Design review of the part built by this model. Coordinates are the model's own, in mm. A direction names the side the tool comes from. Coordinates: 2 decimals unless noted, no trailing zeros. Loops run counter-clockwise (first coordinate to the right, second up) from the corner with the lowest first, then second, coordinate; pieces in that order, holes last. Notation, with made-up numbers: (-40, 81) -> (12, 81) arc R15 cw to (12, 92) -> close; hole circle Ø10 at (79, 66). An arc over 180 degrees is marked (long way). Answer in a Markdown table with one row per item.
Autodesk Inventor part; units mm, degrees
ref_plane "YZ Plane" through (0, 0, 0) normal (1, 0, 0) x (0, 1, 0)
ref_plane "XZ Plane" through (0, 0, 0) normal (0, 1, 0) x (-1, 0, 0)
ref_plane "XY Plane" through (0, 0, 0) normal (0, 0, 1) x (1, 0, 0)
sketch "Sketch8" plane through (0, 0, 0) normal (1, 0, 0) x (0, 1, 0)
  line L0 (0, 15.5) -> (0, 5.5)
  line L1 (0, 5.5) -> (5, 5.5)
  line L2 (5, 5.5) -> (5, -5.5)
  line L3 (5, -5.5) -> (0, -5.5)
  line L4 (0, -5.5) -> (0, -15.5)
  point P0 (0, 0)
  point P1 (5, 0)
  dimension "d39" = 11
  dimension "d40" = 5
  dimension "d41" = 10
  dimension "d42" = 10
contour flange "Contour Flange1" sketch "Sketch8" thickness 1 bend radius 1 width 15 along (1, 0, 0) mid plane no both sides no wall seen from (0, 0, 10.5) lies toward (0, -1, 0) curves L0 L1 L2 L3 L4
bend "Bend1"
corner "Corner1"
equation "\"d29\" = BendReliefWidth"
equation "\"d30\" = BendReliefDepth"
equation "\"d31\" = MinimumRemnant"
equation "\"d32\" = BendRadius"
equation "\"d34\" = BendRadius"
equation "\"d36\" = CornerReliefSize"
equation "\"d37\" = GapSize"
equation "\"d38\" = JacobiRadiusSize"
equation "\"BendRadius\" = Thickness"
equation "\"BendReliefWidth\" = Thickness"
equation "\"BendReliefDepth\" = 0.5 * Thickness"
equation "\"CornerReliefSize\" = 4 * Thickness"
equation "\"MinimumRemnant\" = 2 * Thickness"
equation "\"TransitionRadius\" = BendRadius"
equation "\"JacobiRadiusSize\" = Thickness"
equation "\"GapSize\" = Thickness"
equation "\"d23\" = BendRadius"
properties part number "M18 - Aluminum Bracket" material "Aluminum 6061"
(1) Take a section at D-D on z = -4. Give the boundary of the cut face in (x, y), and give its area (3 significant figures).
Evaluation:
| item | result |
|---|---|
| outline | (0, 3.87) -> (15, 3.87) -> (15, 4.94) -> (0, 4.94) -> close |
| area | 16.1 mm² |
(2) Tool access review of faces 5 (the flat face through (7, 2, 5.5)), 6 (the flat face through (7, 0, -11)), 7 (the cylindrical face through (7.395, 3.715, -4.199)), 8 (the flat face through (7.4, -0.5, -15.5)): name each direction out of +Z, -Z, +X, -X, +Y, -Y from which nothing blocks a thin tool from reaching the whole face with its end or side.
Evaluation:
| item | result |
|---|---|
| face 5 | +Z, +X, -X, +Y |
| face 6 | -Z, +X, -X, +Y |
| face 7 | +X, -X, -Y |
| face 8 | -Z, +X, -X, +Y, -Y |
(3) For pin 1 (2 mm diameter, centred on x = 5.5, z = 1, fed in from -Y); pin 2 (2 mm diameter, centred on x = 6.5, y = 2.5, fed in from -Z); pin 3 (1.5 mm diameter, centred on y = 3.5, z = 3.5, fed in from -X); pin 4 (2 mm diameter, centred on x = 4.5, y = 1.5, fed in from +Z), all flat-tipped, find the tip position at first contact; note any pin that passes through.
Evaluation:
| item | result |
|---|---|
| pin 1 | stops at y = 4 |
| pin 2 | stops at z = -5.5 |
| pin 3 | stops at x = 0 |
| pin 4 | stops at z = 5.63 |
(4) Take a section at B-B on y = 3.6. Give the boundary of the cut face in (x, z).
Evaluation:
| item | result |
|---|---|
| outline | (0, -5.41) -> (15, -5.41) -> (15, -4.3) -> (0, -4.3) -> close; (0, 4.3) -> (15, 4.3) -> (15, 5.41) -> (0, 5.41) -> close |
(5) Take a section at C-C on z = -9.5. Give the boundary of the cut face in (x, y).
Evaluation:
| item | result |
|---|---|
| outline | (0, -1) -> (15, -1) -> (15, 0) -> (0, 0) -> close |
(6) To check wall thickness, follow probe 1 along Z at (x, y) = (7.25, 1.1); probe 2 along Y at (x, z) = (1.25, 13); probe 3 along Y at (x, z) = (6, -2). State the ranges of each line that lie inside material, in increasing order.
Evaluation:
| item | result |
|---|---|
| probe 1 | z = -5.5 to -4.5, 4.5 to 5.5 |
| probe 2 | y = -1 to 0 |
| probe 3 | y = 4 to 5 |
(7) Take a section at A-A on x = 4.5. Give the boundary of the cut face in (y, z), and give its area (3 significant figures).
Evaluation:
| item | result |
|---|---|
| outline | (-1, -15.5) -> (0, -15.5) -> (0, -6.5) arc R1 cw to (1, -5.5) -> (3, -5.5) arc R2 ccw to (5, -3.5) -> (5, 3.5) arc R2 ccw to (3, 5.5) -> (1, 5.5) arc R1 cw to (0, 6.5) -> (0, 15.5) -> (-1, 15.5) -> (-1, 6.5) arc R2 ccw to (1, 4.5) -> (3, 4.5) arc R1 cw to (4, 3.5) -> (4, -3.5) arc R1 cw to (3, -4.5) -> (1, -4.5) arc R2 ccw to (-1, -6.5) -> close |
| area | 38.4 mm² |
(8) Draft analysis for pull direction Z (two halves, no side actions). For faces 1 (the cylindrical face through (7.395, 0.285, -5.801)), 2 (the cylindrical face through (7.4, -0.4, 5.07)), 3 (the flat face through (7, 4, 0)), 4 (the flat face through (15, 4.2, 0.1)), state which applies: pulls with the +Z half, pulls with the -Z half, needs draft (parallel to the pull), parting line crosses it, or undercut.
Evaluation:
| item | result |
|---|---|
| face 1 | pulls with the -Z half |
| face 2 | undercut |
| face 3 | undercut |
| face 4 | needs draft |
